from build123d import *

# Parameters (mm, degrees)
SKETCH3_R               = 1.9812
CUT_EXTRUDE1_DEPTH      = 8.874
CUT_EXTRUDE1_DEPTH_BACK = 8.874


with BuildPart() as part:
    # Sketch2 → Revolve1 (revolve)
    with BuildSketch(Plane(origin=(0, 0, 0), x_dir=(0, 0, -1), z_dir=(1, 0, 0))):
        Polygon((51.562, 6.35), (-48.768, 6.35), (-48.768, 7.874), (-51.816, 7.874), (-52.832, 6.858), (-52.832, 0), (52.832, 0), (52.832, 5.08), align=None)
    revolve(axis=Axis((0, 0, 52.832), (0, 0, -1)))

    # Sketch3 → Cut-Extrude1 (cut, two sides)
    with BuildSketch(Plane(origin=(0, 0, 0), x_dir=(0, 0, -1), z_dir=(1, 0, 0))) as cut_extrude1_sk:
        with Locations((48.860075, 0)):
            Circle(SKETCH3_R)
    extrude(amount=CUT_EXTRUDE1_DEPTH, mode=Mode.SUBTRACT)
    extrude(cut_extrude1_sk.sketch, amount=-CUT_EXTRUDE1_DEPTH_BACK, mode=Mode.SUBTRACT)


solid = part.part
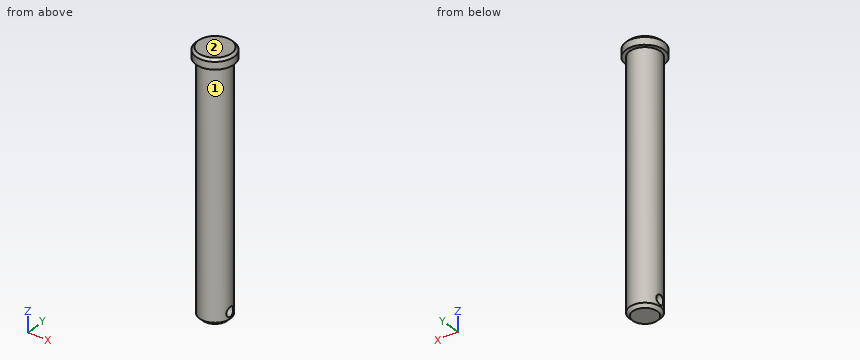
Here's how the part is built. I have some questions about the finished solid (model axes, mm). Face numbers are marked on the shaded views. A direction names the side the tool comes from. Coordinates: 2 decimals unless noted, no trailing zeros. Order: outer loops, then holes, each group sorted by start corner. A loop starts at its lowest first (then second) coordinate and runs counter-clockwise, first axis right, second up. Notation, with made-up numbers: (13, -18) - (17, -18) arc R23 ccw to (17, 0) - close; hole circle Ø7 at (54, -22). An arc over 180 degrees is marked (long way). Use CSV: the item, a comma, the result in double quotes. Start each with the question number.
1. Please list where these lines run through material, in increasing order: line 1 (Y direction, x = -0.5, z = 47); line 2 (X direction, y = -0.25, z = -16); line 3 (Z direction, x = 5, y = 4.5). Write a range as from..to.
2. I'm going to push flat-ended pins straight in: pin 1 (5 mm diameter, centred on y = 3.5, z = -41.5, fed in from -X); pin 2 (5 mm diameter, centred on x = -6, z = 10, fed in from +Y); pin 3 (3 mm diameter, centred on y = -1, z = -7.5, fed in from +X); pin 4 (3.5 mm diameter, centred on y = 0, z = -48.86, fed in from +X). Where does each tip first touch, or does it pass through?
3. For the marked faces 1 and 2, which set-ups out of +Z, -Z, +X, -X, +Y, -Y let a thin tool reach every point of the face, with its end or its side?
4. Suppose I cut it at A-A on y = 0. List the corners of the cut face in (x, z) for me.
5. Suppose I cut it at B-B on z = -44. List the corners of the cut face in (x, y) for me, then the cut area to 3 significant figures.
Output:
1,line 1,"y = -6.33..6.33"
1,line 2,"x = -6.35..6.35"
1,line 3,"z = 48.77..52.83"
2,pin 1,"stops at x = -6.27"
2,pin 2,"stops at y = 5.3"
2,pin 3,"stops at x = 6.35"
2,pin 4,"passes through"
3,face 1,"-Z"
3,face 2,"+Z, +X, -X, +Y, -Y"
4,outline,"(-7.87, 48.77) - (-6.35, 48.77) - (-6.35, -46.88) - (6.35, -46.88) - (6.35, 48.77) - (7.87, 48.77) - (7.87, 51.82) - (6.86, 52.83) - (-6.86, 52.83) - (-7.87, 51.82) - close; (-6.35, -51.56) - (-5.08, -52.83) - (5.08, -52.83) - (6.35, -51.56) - (6.35, -50.84) - (-6.35, -50.84) - close"
5,outline,"circle Ø12.7 at (0, 0)"
5,area,"127 mm2"
